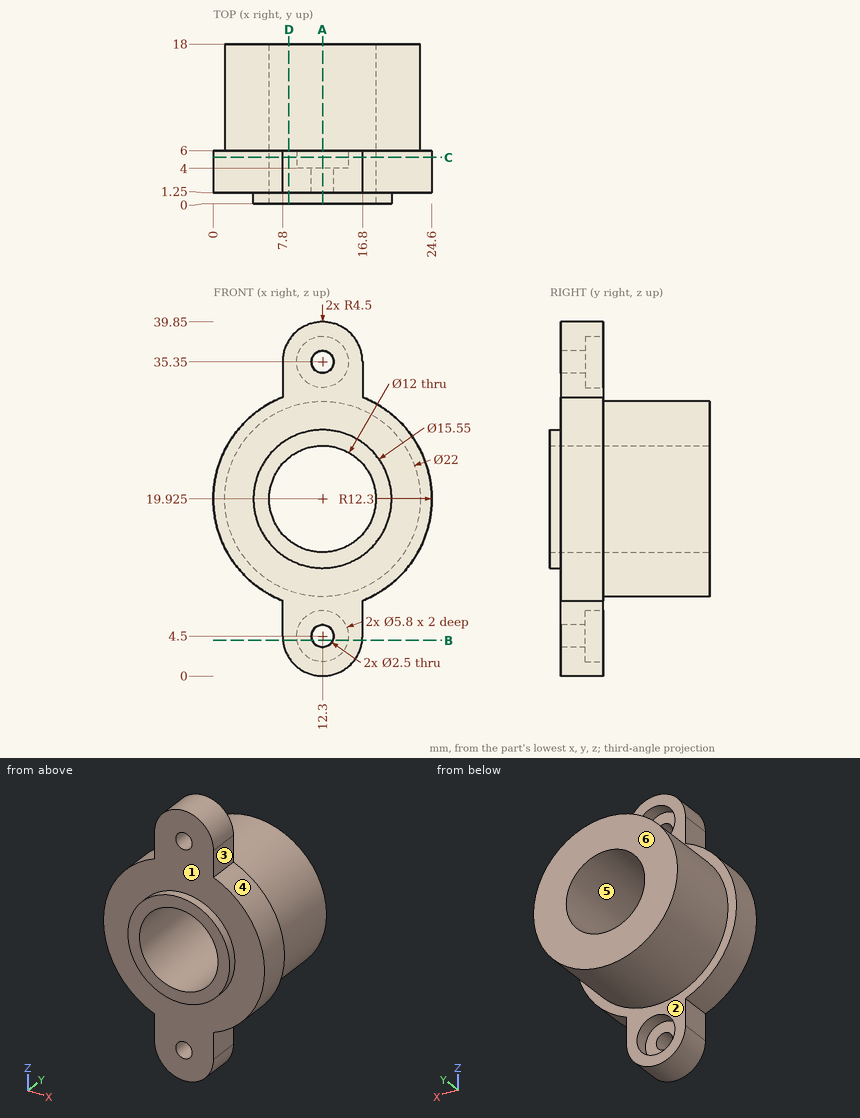
Design review of the part shown in the three views and the two pictorial views. Dimensions are in mm from the part's minimum x, y and z. A direction names the side the tool comes from. Round coordinates to 2 decimals unless told otherwise and drop trailing zeros. Loops run counter-clockwise (first coordinate to the right, second up) from the corner with the lowest first, then second, coordinate; pieces in that order, holes last. Notation, with made-up numbers: (59.5, 10.25) - (68.5, 10.25) arc R22 cw to (68.5, 35.25) - close; hole circle Ø5 at (47.25, 33.5). An arc over 180 degrees is marked (long way). Use one line per item in the form item = value.
1) Wall thickness on probe 1 along Z at (x, y) = (12.3, 5.25) (3 decimals); probe 2 along Z at (x, y) = (12.3, 2.65) (3 decimals); probe 3 along Z at (x, y) = (12.25, 15.25): over which ranges is each line inside the solid? List them lowest first.
Solutions:
probe_1 = 0 to 1.6, 7.4 to 13.925, 25.925 to 32.45, 38.25 to 39.85
probe_2 = 0 to 3.25, 5.75 to 13.925, 25.925 to 34.1, 36.6 to 39.85
probe_3 = 8.93 to 13.93, 25.92 to 30.92
2) We need section B-B on z = 4. Write out the cut boundary in (x, y), then the cut area to 3 significant figures.
Solutions:
outline = (7.83, 1.25) - (11.15, 1.25) - (11.15, 4) - (9.44, 4) - (9.44, 6) - (7.83, 6) - close; (13.45, 1.25) - (16.77, 1.25) - (16.77, 6) - (15.16, 6) - (15.16, 4) - (13.45, 4) - close
area = 24.8 mm2
3) Clearance check with flat-ended pins moving along their axes: P1, Ø10, axis at y = 7, z = 14.5, coming from the -X side; P2, Ø6, axis at y = 10.5, z = 31.5, coming from the +X side; P3, Ø4.5, axis at x = 12.3, z = 35.35, coming from the -Y side; P4, Ø2, axis at x = 12.3, z = 35.35, coming from the +Y side. State where each tip first meets the part, or that it passes through.
Solutions:
P1 = 0.01
P2 = 19.19
P3 = 1.25
P4 = through
4) Mouldability with a two-part tool opening along X and no side actions: class the marked faces 4, 5 and 6 as pulls with the +X half, pulls with the -X half, needs draft (parallel to the pull), parting line crosses it, or undercut.
Solutions:
face_4 = pulls with the +X half
face_5 = undercut
face_6 = needs draft
5) We need section A-A on x = 12.3. State how many separate pieces and enclosed holes the cut face has, then the cut area to 3 significant figures.
Solutions:
separate_pieces = 4
enclosed_holes = 0
area = 220 mm2
6) We need section D-D on x = 8.5. Write out the cut boundary in (y, z).
Solutions:
outline = (0, 13.14) - (1.25, 13.14) - (1.25, 2.09) - (6, 2.09) - (6, 9.6) - (18, 9.6) - (18, 15.28) - (0, 15.28) - close; (0, 24.57) - (18, 24.57) - (18, 30.25) - (6, 30.25) - (6, 37.76) - (1.25, 37.76) - (1.25, 26.71) - (0, 26.71) - close
7) Tool access review of the marked faces 1, 2 and 3: name each direction out of +Z, -Z, +X, -X, +Y, -Y from which nothing blocks a thin tool from reaching the whole face with its end or side.
Solutions:
face_1 = -Y
face_2 = +Y
face_3 = +Z, +X, +Y, -Y
8) We need section C-C on y = 5.25. Write out the cut boundary in (x, z) (3 decimals).
Solutions:
outline = (7.8, 4.5) arc R4.5 ccw to (16.8, 4.5) - (16.8, 8.478) arc R12.3 ccw to (16.8, 31.372) - (16.8, 35.35) arc R4.5 ccw to (7.8, 35.35) - (7.8, 31.372) arc R12.3 ccw to (7.8, 8.478) - close; hole circle Ø12 at (12.3, 19.925); hole circle Ø5.8 at (12.3, 4.5); hole circle Ø5.8 at (12.3, 35.35)
